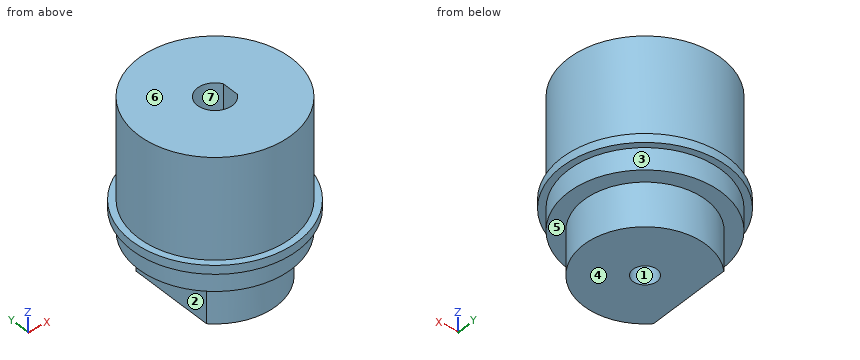
from build123d import *

# Parameters (mm, degrees)
SKETCH1_R           = 14
BOSS_EXTRUDE2_DEPTH = 10
SKETCH2_R           = 17.5
BOSS_EXTRUDE3_DEPTH = 5
SKETCH3_R           = 19
BOSS_EXTRUDE4_DEPTH = 2
SKETCH4_R           = 17.5
BOSS_EXTRUDE5_DEPTH = 23
CUT_EXTRUDE1_DEPTH  = 10
SKETCH10_R          = 2.75
CUT_EXTRUDE2_DEPTH  = 15
CUT_EXTRUDE3_DEPTH  = 15


with BuildPart() as part:
    # Sketch1 → Boss-Extrude2 (new body)
    with BuildSketch(Plane.XY):
        Circle(SKETCH1_R)
    extrude(amount=BOSS_EXTRUDE2_DEPTH)

    # Sketch2 → Boss-Extrude3 (add)
    with BuildSketch(Plane.XY.offset(10)):
        Circle(SKETCH2_R)
    extrude(amount=BOSS_EXTRUDE3_DEPTH)

    # Sketch3 → Boss-Extrude4 (add)
    with BuildSketch(Plane.XY.offset(15)):
        Circle(SKETCH3_R)
    extrude(amount=BOSS_EXTRUDE4_DEPTH)

    # Sketch4 → Boss-Extrude5 (add)
    with BuildSketch(Plane.XY.offset(17)):
        Circle(SKETCH4_R)
    extrude(amount=BOSS_EXTRUDE5_DEPTH)

    # Sketch5 → Cut-Extrude1 (cut)
    with BuildSketch(Plane(origin=(0, 0, 0), x_dir=(-1, 0, 0), z_dir=(0, 0, -1))):
        with BuildLine():
            Line((10, 0), (10, -9.797958971))
            ThreePointArc((10, -9.797958971), (14, 0), (10, 9.797958971))
            Line((10, 9.797958971), (10, 0))
        make_face()
    extrude(amount=-CUT_EXTRUDE1_DEPTH, mode=Mode.SUBTRACT)

    # Sketch10 → Cut-Extrude2 (cut)
    with BuildSketch(Plane(origin=(0, 0, 0), x_dir=(-1, 0, 0), z_dir=(0, 0, -1))):
        Circle(SKETCH10_R)
    extrude(amount=-CUT_EXTRUDE2_DEPTH, mode=Mode.SUBTRACT)

    # Sketch12 → Cut-Extrude3 (cut)
    with BuildSketch(Plane.XY.offset(40)):
        with BuildLine():
            Line((3.5, 0), (3.5, -1.936491673))
            ThreePointArc((3.5, -1.936491673), (-4, 0), (3.5, 1.936491673))
            Line((3.5, 1.936491673), (3.5, 0))
        make_face()
    extrude(amount=-CUT_EXTRUDE3_DEPTH, mode=Mode.SUBTRACT)


solid = part.part
Here's how the part is built. I have some questions about the finished solid (model axes, mm). Face numbers are marked on the shaded views. A direction names the side the tool comes from. Give positions to 0.01 mm unless a question says otherwise; leave off trailing zeros. Order: outer loops, then holes, each group sorted by start corner. A loop starts at its lowest first (then second) coordinate and runs counter-clockwise, first axis right, second up. Notation, with made-up numbers: (31.25, 47) -> (70.25, 47) arc R29 cw to (70.25, 78) -> close; hole circle Ø5 at (-19.5, 21). An arc over 180 degrees is marked (long way). Use a Markdown table: item, result. Add a question column.
Item 1: For the marked faces 5, 6 and 7, which set-ups out of +Z, -Z, +X, -X, +Y, -Y let a thin tool reach every point of the face, with its end or its side?
Item 2: If we mould it in two halves opening along X, with no side actions, what happens to the marked faces 1, 2, 3 and 4? For each: pulls with the +X half, pulls with the -X half, needs draft (parallel to the pull), parting line crosses it, or undercut.
Item 3: Imagine slicing it at D-D on z = 21. Please give me the cut outline in (x, y).
Item 4: I need wall thicknesses on line 1 (Y direction, x = 0, z = 28.5); line 2 (Y direction, x = 0, z = 11); line 3 (Z direction, x = -5, y = 14). Which ranges of each line are inside material? Lowest first, please.
Item 5: Imagine slicing it at B-B on x = 0. Please give me the cut outline in (y, z).
Item 6: Imagine slicing it at C-C on z = 37. Please give me the cut outline in (x, y), plus the area to 3 significant figures.
Item 7: Will these pins go through, and if not, where does the flat tip stop? pin 1 (6.5 mm diameter, centred on x = 0, y = 0, fed in from +Z); pin 2 (12 mm diameter, centred on y = -8.5, z = 15, fed in from -X); pin 3 (1.9 mm diameter, centred on y = 0, z = 29, fed in from -X).
Item 8: Imagine slicing it at A-A on y = 0. Please give me the cut outline in (x, z).
Data:
| question | item | result |
|---|---|---|
| 1 | face 5 | -Z |
| 1 | face 6 | +Z, +X, -X, +Y, -Y |
| 1 | face 7 | +Z |
| 2 | face 1 | undercut |
| 2 | face 2 | pulls with the -X half |
| 2 | face 3 | parting line crosses it |
| 2 | face 4 | needs draft |
| 3 | outline | circle Ø35 at (0, 0) |
| 4 | line 1 | y = -17.5 to -4, 4 to 17.5 |
| 4 | line 2 | y = -17.5 to -2.75, 2.75 to 17.5 |
| 4 | line 3 | z = 10 to 40 |
| 5 | outline | (-19, 15) -> (-17.5, 15) -> (-17.5, 10) -> (-14, 10) -> (-14, 0) -> (-2.75, 0) -> (-2.75, 15) -> (2.75, 15) -> (2.75, 0) -> (14, 0) -> (14, 10) -> (17.5, 10) -> (17.5, 15) -> (19, 15) -> (19, 17) -> (17.5, 17) -> (17.5, 40) -> (4, 40) -> (4, 25) -> (-4, 25) -> (-4, 40) -> (-17.5, 40) -> (-17.5, 17) -> (-19, 17) -> close |
| 6 | outline | circle Ø35 at (0, 0); hole (3.5, -1.94) -> (3.5, 1.94) arc R4 ccw (long way) to start |
| 6 | area | 913 mm² |
| 7 | pin 1 | stops at z = 25 |
| 7 | pin 2 | stops at x = -18.83 |
| 7 | pin 3 | stops at x = -17.5 |
| 8 | outline | (-19, 15) -> (-17.5, 15) -> (-17.5, 10) -> (-10, 10) -> (-10, 0) -> (-2.75, 0) -> (-2.75, 15) -> (2.75, 15) -> (2.75, 0) -> (14, 0) -> (14, 10) -> (17.5, 10) -> (17.5, 15) -> (19, 15) -> (19, 17) -> (17.5, 17) -> (17.5, 40) -> (3.5, 40) -> (3.5, 25) -> (-4, 25) -> (-4, 40) -> (-17.5, 40) -> (-17.5, 17) -> (-19, 17) -> close |
